from build123d import *

# Parameters (mm, degrees)
SKETCH1_W                     = 292.1
SKETCH1_H                     = 76.2
SKETCH1_R                     = 3.96875
BOSS_EXTRUDE1_DEPTH           = 6.35
MASTER_CYLINDER_OPENING_REACH = 8.35
SKETCH2_W                     = 83.82
SKETCH2_H                     = 19.05


with BuildPart() as part:
    # Sketch1 → Boss-Extrude1 (new body)
    with BuildSketch(Plane(origin=(0, 0, 0), x_dir=(1, 0, 0), z_dir=(0, 1, 0))):
        with Locations((146.05, 38.1)):
            Rectangle(SKETCH1_W, SKETCH1_H)
        with Locations((12.7, 63.5)):
            Circle(SKETCH1_R, mode=Mode.SUBTRACT)
        with Locations((12.7, 38.1)):
            Circle(SKETCH1_R, mode=Mode.SUBTRACT)
        with Locations((12.7, 12.7)):
            Circle(SKETCH1_R, mode=Mode.SUBTRACT)
        with Locations((279.4, 12.7)):
            Circle(SKETCH1_R, mode=Mode.SUBTRACT)
        with Locations((279.4, 38.1)):
            Circle(SKETCH1_R, mode=Mode.SUBTRACT)
        with Locations((279.4, 63.5)):
            Circle(SKETCH1_R, mode=Mode.SUBTRACT)
    extrude(amount=BOSS_EXTRUDE1_DEPTH)

    # Sketch2 → Master Cylinder Opening (cut, up to next)
    with BuildSketch(Plane(origin=(0, 6.35, 0), x_dir=(1, 0, 0), z_dir=(0, 1, 0)), mode=Mode.PRIVATE) as master_cylinder_opening_sk1:
        with Locations((146.05, 66.675)):
            Rectangle(SKETCH2_W, SKETCH2_H)
    master_cylinder_opening_tool1 = extrude(master_cylinder_opening_sk1.sketch, amount=-MASTER_CYLINDER_OPENING_REACH, mode=Mode.PRIVATE) & part.part
    add(master_cylinder_opening_tool1.solids().sort_by_distance((146.05, 6.35, -66.675))[0], mode=Mode.SUBTRACT)


solid = part.part
The model under review builds one solid part; all positions refer to its coordinate system, in mm. A direction names the side the tool comes from. Coordinates: 2 decimals unless noted, no trailing zeros. Write each loop counter-clockwise with the first axis right and the second up, starting at its lowest first coordinate (ties: lowest second). Pieces come first, ordered by that corner, then holes. Notation, with made-up numbers: (20.25, 17.25) -> (50.25, 17.25) arc R22 cw to (50.25, 31.25) -> close; hole circle Ø1 at (30.5, 38). An arc over 180 degrees is marked (long way). Answer in a Markdown table with one row per item.
1. For faces 1 (the flat face through (144, 6.35, -39)), 2 (the flat face through (145, 3, -57.15)), list the 3-axis set-ups (+Z, -Z, +X, -X, +Y, -Y) from which the entire face can be reached by the end or side of a thin tool; tool diameter is ignored.
Answers below:
| item | result |
|---|---|
| face 1 | +Z, -Z, +X, -X, +Y |
| face 2 | -Z, +Y, -Y |
2. Draft analysis for pull direction Z (two halves, no side actions). For faces 3 (the flat face through (51, 3, -76.2)), 4 (the cylindrical face through (8.735, 3.131, -12.874)), 5 (the cylindrical face through (283.185, 3.131, -64.692)), 6 (the flat face through (292.1, 3, -38)), state which applies: +Z half, -Z half, draft (parallel to the pull), parting line (faces both ways), or undercut.
Answers below:
| item | result |
|---|---|
| face 3 | -Z half |
| face 4 | undercut |
| face 5 | undercut |
| face 6 | draft |
3. We need section B-B, the plane x = 279.4. State the section outline as (y, z) points.
Answers below:
| item | result |
|---|---|
| outline | (0, -76.2) -> (6.35, -76.2) -> (6.35, -67.47) -> (0, -67.47) -> close; (0, -59.53) -> (6.35, -59.53) -> (6.35, -42.07) -> (0, -42.07) -> close; (0, -34.13) -> (6.35, -34.13) -> (6.35, -16.67) -> (0, -16.67) -> close; (0, -8.73) -> (6.35, -8.73) -> (6.35, 0) -> (0, 0) -> close |
4. Clearance check with flat-ended pins moving along their axes: pin 1 Ø6.5 at (x, z) = (12.7, -12.7) entering from -Y; pin 2 Ø3 at (x, y) = (152.5, 3) entering from -Z. State where each tip first meets the part, or that it passes through.
Answers below:
| item | result |
|---|---|
| pin 1 | passes through |
| pin 2 | stops at z = -57.15 |
5. We need section D-D, the plane y = 3. State the section outline as (x, z) points, and give its area (3 significant figures).
Answers below:
| item | result |
|---|---|
| outline | (0, -76.2) -> (104.14, -76.2) -> (104.14, -57.15) -> (187.96, -57.15) -> (187.96, -76.2) -> (292.1, -76.2) -> (292.1, 0) -> (0, 0) -> close; hole circle Ø7.94 at (12.7, -63.5); hole circle Ø7.94 at (12.7, -38.1); hole circle Ø7.94 at (12.7, -12.7); hole circle Ø7.94 at (279.4, -63.5); hole circle Ø7.94 at (279.4, -38.1); hole circle Ø7.94 at (279.4, -12.7) |
| area | 20,400 mm^2 |
6. We need section C-C, the plane z = -63.5. State the section outline as (x, y) points, and give its area (3 significant figures).
Answers below:
| item | result |
|---|---|
| outline | (0, 0) -> (8.73, 0) -> (8.73, 6.35) -> (0, 6.35) -> close; (16.67, 0) -> (104.14, 0) -> (104.14, 6.35) -> (16.67, 6.35) -> close; (187.96, 0) -> (275.43, 0) -> (275.43, 6.35) -> (187.96, 6.35) -> close; (283.37, 0) -> (292.1, 0) -> (292.1, 6.35) -> (283.37, 6.35) -> close |
| area | 1,220 mm^2 |
7. We need section A-A, the plane z = -38.1. State the section outline as (x, y) points.
Answers below:
| item | result |
|---|---|
| outline | (0, 0) -> (8.73, 0) -> (8.73, 6.35) -> (0, 6.35) -> close; (16.67, 0) -> (275.43, 0) -> (275.43, 6.35) -> (16.67, 6.35) -> close; (283.37, 0) -> (292.1, 0) -> (292.1, 6.35) -> (283.37, 6.35) -> close |
8. Wall thickness on probe 1 along Z at (x, y) = (12.7, 5.25); probe 2 along Z at (x, y) = (280, 5.5); probe 3 along X at (y, z) = (4.5, -68.5): over which ranges is each line inside the solid? List them lowest first. Write a range as [from, to].
Answers below:
| item | result |
|---|---|
| probe 1 | z = [-76.2, -67.47], [-59.53, -42.07], [-34.13, -16.67], [-8.73, 0] |
| probe 2 | z = [-76.2, -67.42], [-59.58, -42.02], [-34.18, -16.62], [-8.78, 0] |
| probe 3 | x = [0, 104.14], [187.96, 292.1] |
